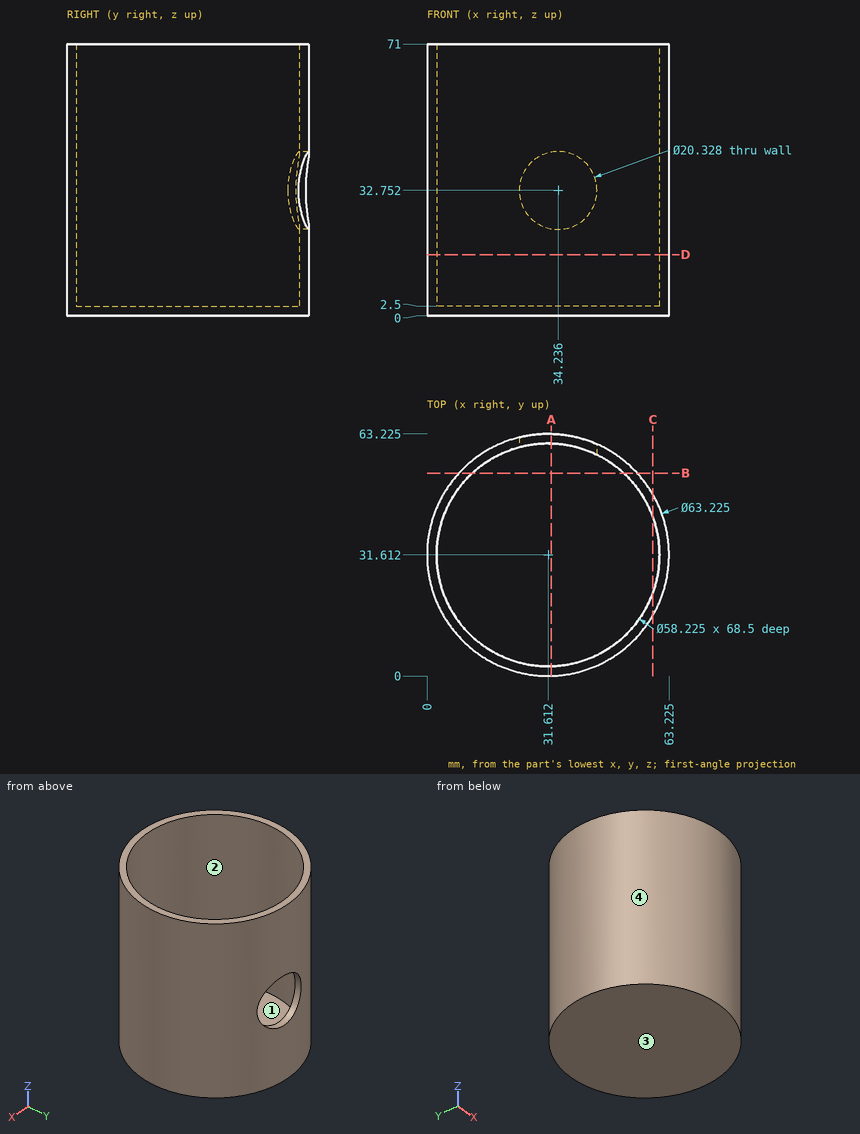
Part print with two shaded views. Sizes in mm from the minimum x, y, z corner. Round coordinates to 2 decimals unless told otherwise and drop trailing zeros. Loops run counter-clockwise (first coordinate to the right, second up) from the corner with the lowest first, then second, coordinate; pieces in that order, holes last.
Item 1: Saw through at D-D (z = 16). List the corners of the cut face in (x, y) (1 decimal), then the cut area to 3 significant figures.
Item 2: Pin check, flat tips, straight feed: P1, Ø16.5, axis at x = 34.24, z = 32.75, coming from the -Y side; P2, Ø1, axis at y = 53, z = 37.5, coming from the -X side (1 decimal); P3, Ø4, axis at x = 22.5, z = 49.5, coming from the +Y side (1 decimal). Stop position of each tip, or through.
Item 3: Saw through at A-A (x = 32.5). List the corners of the cut face in (y, z).
Item 4: Saw through at B-B (y = 53). List the corners of the cut face in (x, z).
Item 5: Saw through at C-C (x = 59). List the corners of the cut face in (y, z) (1 decimal).
Item 6: Two-plate mould, pull along Y, no slides. Class the marked faces 1, 2, 3 and 4: released by +Y, released by -Y, zero draft, split by the parting line, or undercut.
Item 7: Drill centre lines: line 1 along Y through (x, z) = (30.5, 45) (1 decimal); line 2 along Z through (x, y) = (42.5, 18); line 3 along X through (y, z) = (27.5, 21). Where is each one in solid material? Low to high.
Worked answers:
1. outline: circle Ø63.2 at (31.6, 31.6); hole circle Ø58.2 at (31.6, 31.6)
1. area: 477 mm2
2. P1: stops at y = 0
2. P2: stops at x = 7.9
2. P3: stops at y = 62.4
3. outline: (0.01, 0) - (63.21, 0) - (63.21, 22.74) - (60.71, 22.74) - (60.71, 2.5) - (2.51, 2.5) - (2.51, 71) - (0.01, 71) - close; (60.71, 42.77) - (63.21, 42.77) - (63.21, 71) - (60.71, 71) - close
4. outline: (8.33, 0) - (54.89, 0) - (54.89, 71) - (51.36, 71) - (51.36, 2.5) - (11.86, 2.5) - (11.86, 71) - (8.33, 71) - close
5. outline: (15.8, 0) - (47.4, 0) - (47.4, 71) - (41.5, 71) - (41.5, 2.5) - (21.7, 2.5) - (21.7, 71) - (15.8, 71) - close
6. face 1: undercut
6. face 2: undercut
6. face 3: zero draft
6. face 4: split by the parting line
7. line 1: y = 0 to 2.5, 60.7 to 63.2
7. line 2: z = 0 to 2.5
7. line 3: x = 0.27 to 2.79, 60.43 to 62.96
